Can you work these out from the model? Positions are in its coordinate system, mm. A direction names the side the tool comes from. Round coordinates to 2 decimals unless told otherwise and drop trailing zeros. Write each loop counter-clockwise with the first axis right and the second up, starting at its lowest first coordinate (ties: lowest second). Pieces come first, ordered by that corner, then holes.
Q1. If we section it at B-B (z = -8.5): Please give me the cut outline in (x, y).
Q2. For faces 4 (the cylindrical face through (-5.723, -1.802, -14.253)), 5 (the cylindrical face through (0.867, 3.905, -21.042)), 6 (the flat face through (3, 4, -10.4)), 7 (the flat face through (-4, -4, 0)), which set-ups out of +Z, -Z, +X, -X, +Y, -Y let a thin tool reach every point of the face, with its end or its side?
Q3. We'd pull the mould along Z, two halves only. Please class faces 1 (the cylindrical face through (-5.723, -1.802, -4.056)), 2 (the flat face through (-3, 4, -8)), 3 (the flat face through (1.42, 3.92, -18)): +Z half, -Z half, draft (parallel to the pull), parting line (faces both ways), or undercut.
Q4. If we section it at A-A (z = -5.5): Please give me the cut outline in (x, y).
Q5. Please list where these lines run through material, in increasing order: line 1 along Z through (x, y) = (5, -2); line 2 along X through (y, z) = (3, -16); line 3 along Y through (x, z) = (3.75, -16.75).
Q6. I'm going to push flat-ended pins straight in: pin 1 Ø3.5 at (x, y) = (2, -0.5) entering from +Z; pin 2 Ø6 at (y, z) = (-3.5, -15) entering from -X; pin 3 Ø1 at (y, z) = (-1, -18) entering from +X. Where does each tip first touch, or does it pass through?
from build123d import *


with BuildPart() as part:
    # 草图1 → 旋转1 (revolve)
    with BuildSketch(Plane(origin=(0, 0, 0), x_dir=(1, 0, 0), z_dir=(0, 1, 0)), mode=Mode.PRIVATE) as revolve_1_sk:
        with BuildLine():
            Line((5, 0), (6, 0))
            Line((6, 0), (6, 8))
            Line((6, 8), (4.3, 8))
            Line((4.3, 8), (4.3, 10.4))
            Line((4.3, 10.4), (6, 10.4))
            Line((6, 10.4), (6, 18))
            Line((6, 18), (4, 18))
            Line((4, 18), (4, 24))
            Line((4, 24), (0, 24))
            Line((0, 24), (0, -5))
            ThreePointArc((0, -5), (3.5355, -3.5355), (5, 0))
        make_face()
    revolve(revolve_1_sk.sketch.rotate(Axis((0, 0, -30), (0, 0, 1)), 180), axis=Axis((0, 0, -30), (0, 0, 1)))


solid = part.part
A:
1. outline: circle Ø8.6 at (0, 0)
2. face 4: +Z, -Z
2. face 5: -Z
2. face 6: none
2. face 7: +Z
3. face 1: draft
3. face 2: undercut
3. face 3: -Z half
4. outline: circle Ø12 at (0, 0)
5. line 1: z = -18 to -10.4, -8 to 0
5. line 2: x = -5.2 to 5.2
5. line 3: y = -4.68 to 4.68
6. pin 1: stops at z = 4.99
6. pin 2: stops at x = -5.98
6. pin 3: stops at x = 5.98
